Design review of the part built by this model. Coordinates are the model's own, in mm. A direction names the side the tool comes from. Coordinates: 2 decimals unless noted, no trailing zeros. Order: outer loops, then holes, each group sorted by start corner. A loop starts at its lowest first (then second) coordinate and runs counter-clockwise, first axis right, second up.
from build123d import *

# Parameters (mm, degrees)
SKETCH1_W           = 90
SKETCH1_H           = 90
BOSS_EXTRUDE1_DEPTH = 10
CUT_EXTRUDE1_DEPTH  = 6.9
SKETCH3_R           = 1.5
CUT_EXTRUDE2_DEPTH  = 11
SKETCH4_R           = 5
CUT_EXTRUDE3_DEPTH  = 11
CUT_EXTRUDE4_DEPTH  = 6.9
FILLET1_R           = 5


with BuildPart() as part:
    # Sketch1 → Boss-Extrude1 (new body)
    with BuildSketch(Plane(origin=(0, 0, 0), x_dir=(1, 0, 0), z_dir=(0, 1, 0))):
        Rectangle(SKETCH1_W, SKETCH1_H)
    extrude(amount=BOSS_EXTRUDE1_DEPTH)

    # Sketch2 → Cut-Extrude1 (cut)
    with BuildSketch(Plane.XZ):
        Polygon((-4.618802154, -8), (4.618802154, -8), (9.237604307, 0), (4.618802154, 8), (-4.618802154, 8), (-9.237604307, 0), align=None)
        with BuildLine():
            Line((-8.754828956, 15.286801604), (-12.02081528, 12.02081528))
            ThreePointArc((-12.02081528, 12.02081528), (12.02081528, 12.02081528), (12.02081528, -12.02081528))
            Line((12.02081528, -12.02081528), (15.286801604, -8.754828956))
            Line((15.286801604, -8.754828956), (24.209642177, -11.145696882))
            Line((24.209642177, -11.145696882), (26.494591989, -19.673245674))
            ThreePointArc((26.494591989, -19.673245674), (23.334523779, 23.334523779), (-19.673245674, 26.494591989))
            Line((-19.673245674, 26.494591989), (-11.145696882, 24.209642177))
            Line((-11.145696882, 24.209642177), (-8.754828956, 15.286801604))
        make_face()
        with BuildLine():
            Line((15.286801604, -8.754828956), (12.02081528, -12.02081528))
            ThreePointArc((12.02081528, -12.02081528), (9.950262871, -15.607117349), (9.950263016, -19.74822225))
            ThreePointArc((9.950263016, -19.74822225), (12.020815311, -23.33452381), (15.607116893, -25.405076066))
            ThreePointArc((15.607116893, -25.405076066), (19.748221753, -25.405076177), (23.334523779, -23.334523779))
            ThreePointArc((23.334523779, -23.334523779), (24.981721996, -21.561854422), (26.494591989, -19.673245674))
            Line((26.494591989, -19.673245674), (24.209642177, -11.145696882))
            Line((24.209642177, -11.145696882), (15.286801604, -8.754828956))
        make_face()
        with BuildLine():
            ThreePointArc((-19.748221967, 9.95026294), (-15.607117207, 9.950262909), (-12.02081528, 12.02081528))
            Line((-12.02081528, 12.02081528), (-8.754828956, 15.286801604))
            Line((-8.754828956, 15.286801604), (-11.145696882, 24.209642177))
            Line((-11.145696882, 24.209642177), (-19.673245674, 26.494591989))
            ThreePointArc((-19.673245674, 26.494591989), (-21.561854422, 24.981721996), (-23.334523779, 23.334523779))
            ThreePointArc((-23.334523779, 23.334523779), (-25.405076135, 19.748221911), (-25.405076151, 15.607117209))
            ThreePointArc((-25.405076151, 15.607117209), (-23.334523822, 12.020815323), (-19.748221967, 9.95026294))
        make_face()
        with BuildLine():
            Line((-26.600510103, 20.068537455), (-25.405076151, 15.607117209))
            ThreePointArc((-25.405076151, 15.607117209), (-25.405076135, 19.748221911), (-23.334523779, 23.334523779))
            Line((-23.334523779, 23.334523779), (-26.600510103, 20.068537455))
        make_face()
        with BuildLine():
            Line((-19.748221967, 9.95026294), (-15.286801604, 8.754828956))
            Line((-15.286801604, 8.754828956), (-12.02081528, 12.02081528))
            ThreePointArc((-12.02081528, 12.02081528), (-15.607117207, 9.950262909), (-19.748221967, 9.95026294))
        make_face()
        with BuildLine():
            Line((-24.209642177, 11.145696882), (-19.748221967, 9.95026294))
            ThreePointArc((-19.748221967, 9.95026294), (-23.334523822, 12.020815323), (-25.405076151, 15.607117209))
            Line((-25.405076151, 15.607117209), (-24.209642177, 11.145696882))
        make_face()
        with BuildLine():
            ThreePointArc((9.950263016, -19.74822225), (9.950262871, -15.607117349), (12.02081528, -12.02081528))
            Line((12.02081528, -12.02081528), (8.754828956, -15.286801604))
            Line((8.754828956, -15.286801604), (9.950263016, -19.74822225))
        make_face()
        with BuildLine():
            ThreePointArc((15.607116893, -25.405076066), (12.020815311, -23.33452381), (9.950263016, -19.74822225))
            Line((9.950263016, -19.74822225), (11.145696882, -24.209642177))
            Line((11.145696882, -24.209642177), (15.607116893, -25.405076066))
        make_face()
        with BuildLine():
            ThreePointArc((23.334523779, -23.334523779), (19.748221753, -25.405076177), (15.607116893, -25.405076066))
            Line((15.607116893, -25.405076066), (20.068537455, -26.600510103))
            Line((20.068537455, -26.600510103), (23.334523779, -23.334523779))
        make_face()
    extrude(amount=-CUT_EXTRUDE1_DEPTH, mode=Mode.SUBTRACT)

    # Sketch3 → Cut-Extrude2 (cut, through all)
    with BuildSketch(Plane(origin=(0, 10, 0), x_dir=(1, 0, 0), z_dir=(0, 1, 0))):
        with Locations((-40, 40)):
            Circle(SKETCH3_R)
        with Locations((40, 40)):
            Circle(SKETCH3_R)
        with Locations((40, -40)):
            Circle(SKETCH3_R)
        with Locations((-40, -40)):
            Circle(SKETCH3_R)
    extrude(amount=-CUT_EXTRUDE2_DEPTH, mode=Mode.SUBTRACT)

    # Sketch4 → Cut-Extrude3 (cut, through all)
    with BuildSketch(Plane(origin=(0, 10, 0), x_dir=(1, 0, 0), z_dir=(0, 1, 0))):
        with Locations((-30, 30)):
            Circle(SKETCH4_R)
        with Locations((30, 30)):
            Circle(SKETCH4_R)
        with Locations((30, -30)):
            Circle(SKETCH4_R)
        with Locations((-30, -30)):
            Circle(SKETCH4_R)
    extrude(amount=-CUT_EXTRUDE3_DEPTH, mode=Mode.SUBTRACT)

    # Sketch6 → Cut-Extrude4 (cut)
    with BuildSketch(Plane.XZ):
        Polygon((-25.381197846, 22), (-20.762395693, 30), (-25.381197846, 38), (-34.618802154, 38), (-39.237604307, 30), (-34.618802154, 22), align=None)
        Polygon((34.618802154, 22), (39.237604307, 30), (34.618802154, 38), (25.381197846, 38), (20.762395693, 30), (25.381197846, 22), align=None)
        Polygon((34.618802154, -38), (39.237604307, -30), (34.618802154, -22), (25.381197846, -22), (20.762395693, -30), (25.381197846, -38), align=None)
        Polygon((-20.762395693, -30), (-25.381197846, -22), (-34.618802154, -22), (-39.237604307, -30), (-34.618802154, -38), (-25.381197846, -38), align=None)
    extrude(amount=-CUT_EXTRUDE4_DEPTH, mode=Mode.SUBTRACT)

    # Fillet1
    fillet1_edges = [part.edges().sort_by_distance(p)[0] for p in [
        (45, 5, 45),
        (-45, 5, 45),
        (-45, 5, -45),
        (45, 5, -45),
    ]]
    fillet(fillet1_edges, radius=FILLET1_R)


solid = part.part
1. Mouldability with a two-part tool opening along Z and no side actions: class faces 3 (the flat face through (-13.68, 3.4, 10.36)), 4 (the flat face through (-1, 5, 45)), 5 (the flat face through (-45, 5, 1)) as pulls with the +Z half, pulls with the -Z half, needs draft (parallel to the pull), parting line crosses it, or undercut.
2. To check wall thickness, follow line 1 (Z direction, x = 30, y = 7.6); line 2 (Z direction, x = 40, y = 7.75). State the ranges of each line that lie inside material, in increasing order.
3. Add section B-B (x = -30). Give the boundary of the cut face in (y, z).
4. Insertion check: pin 1 (8 mm diameter, centred on x = 30, z = 30, fed in from +Y); pin 2 (5 mm diameter, centred on x = -1, z = -2, fed in from -Y). Each pin has a flat end and moves straight along its axis. Give the tip position at first contact, or say it passes through.
5. Add section A-A (y = 8). State how many separate pieces and enclosed holes the cut face has, and give its area (3 significant figures).
6. Add section C-C (z = 5). Give the boundary of the cut face in (x, y).
7. For faces 1 (the cylindrical face through (43, 5, 44)), 2 (the flat face through (10.41, 3.4, -13.63)), list the 3-axis set-ups (+Z, -Z, +X, -X, +Y, -Y) from which the entire face can be reached by the end or side of a thin tool; tool diameter is ignored.
8. Add section D-D (x = -1). Give the boundary of the cut face in (y, z), and give its area (3 significant figures).
Solution:
1. face 3: undercut
1. face 4: pulls with the +Z half
1. face 5: needs draft
2. line 1: z = -45 to -35, -25 to 25, 35 to 45
2. line 2: z = -45 to -41.5, -38.5 to 38.5, 41.5 to 45
3. outline: (0, -45) - (10, -45) - (10, -35) - (6.9, -35) - (6.9, -38) - (0, -38) - close; (0, -22) - (6.9, -22) - (6.9, -25) - (10, -25) - (10, 25) - (6.9, 25) - (6.9, 22) - (0, 22) - close; (0, 38) - (6.9, 38) - (6.9, 35) - (10, 35) - (10, 45) - (0, 45) - close
4. pin 1: passes through
4. pin 2: stops at y = 6.9
5. separate pieces: 1
5. enclosed holes: 8
5. area: 7,740 mm2
6. outline: (-45, 0) - (-6.35, 0) - (-6.35, 6.9) - (6.35, 6.9) - (6.35, 0) - (16.25, 0) - (16.25, 6.9) - (32.62, 6.9) - (32.62, 0) - (45, 0) - (45, 10) - (-45, 10) - close
7. face 1: +Z, +X, +Y, -Y
7. face 2: -Y
8. outline: (0, -45) - (10, -45) - (10, 45) - (0, 45) - (0, 32.98) - (6.9, 32.98) - (6.9, 16.97) - (0, 16.97) - (0, 8) - (6.9, 8) - (6.9, -8) - (0, -8) - close
8. area: 679 mm2
